```python
from build123d import *

# Parameters (mm, degrees)
F0_W      = 10
F0_H      = 14
F1_DEPTH  = 3
F2_W      = 7
F2_H      = 28
F3_DEPTH  = 35.5
F5_DEPTH  = 70.001
F6_R      = 11.075
F7_DEPTH  = 7
F9_DEPTH  = 25
F10_R     = 2
F11_DEPTH = 2


with BuildPart() as f1:
    # F0 (on Top) → F1 (new body)
    with BuildSketch(Plane.XY):
        with BuildLine():
            ThreePointArc((25, 23), (24.4142135624, 24.4142135624), (23, 25))
            Line((23, 25), (-23, 25))
            ThreePointArc((-23, 25), (-24.4142135624, 24.4142135624), (-25, 23))
            Line((-25, 23), (-25, 14))
            Line((-25, 14), (-25, 0))
            Line((-25, 0), (-25, -14))
            Line((-25, -14), (-25, -23))
            ThreePointArc((-25, -23), (-24.4142135624, -24.4142135624), (-23, -25))
            Line((-23, -25), (23, -25))
            ThreePointArc((23, -25), (24.4142135624, -24.4142135624), (25, -23))
            Line((25, -23), (25, -14))
            Line((25, -14), (25, 0))
            Line((25, 0), (25, 14))
            Line((25, 14), (25, 23))
        make_face()
        with BuildLine():
            ThreePointArc((-20, 18.4), (-21.1313708499, 21.1313708499), (-18.4, 20))
            Line((-18.4, 20), (18.4, 20))
            ThreePointArc((18.4, 20), (20, 21.6), (21.6, 20))
            ThreePointArc((21.6, 20), (21.1313708499, 18.8686291501), (20, 18.4))
            Line((20, 18.4), (20, -18.4))
            ThreePointArc((20, -18.4), (21.1313708499, -18.8686291501), (21.6, -20))
            ThreePointArc((21.6, -20), (20, -21.6), (18.4, -20))
            Line((18.4, -20), (-18.4, -20))
            ThreePointArc((-18.4, -20), (-21.1313708499, -21.1313708499), (-20, -18.4))
            Line((-20, -18.4), (-20, 18.4))
        make_face(mode=Mode.SUBTRACT)
        with Locations((30, 7)):
            Rectangle(F0_W, F0_H)
        with Locations((-30, 7)):
            Rectangle(F0_W, F0_H)
        with Locations((30, -7)):
            Rectangle(F0_W, F0_H)
        with Locations((-30, -7)):
            Rectangle(F0_W, F0_H)
        with BuildLine():
            Line((18.4, 20), (-18.4, 20))
            ThreePointArc((-18.4, 20), (-18.8686291501, 18.8686291501), (-20, 18.4))
            Line((-20, 18.4), (-20, -18.4))
            ThreePointArc((-20, -18.4), (-18.8686291501, -18.8686291501), (-18.4, -20))
            Line((-18.4, -20), (18.4, -20))
            ThreePointArc((18.4, -20), (18.8686291501, -18.8686291501), (20, -18.4))
            Line((20, -18.4), (20, 18.4))
            ThreePointArc((20, 18.4), (18.8686291501, 18.8686291501), (18.4, 20))
        make_face()
    extrude(amount=F1_DEPTH)

    # F2 (on face) → F3 (join)
    with BuildSketch(Plane.XY.offset(3)):
        with Locations((-31.5, 0)):
            Rectangle(F2_W, F2_H)
        with Locations((31.5, 0)):
            Rectangle(F2_W, F2_H)
    extrude(amount=F3_DEPTH)

    # F4 (on face) → F5 (cut, through all)
    with BuildSketch(Plane(origin=(-35, 0, 0), x_dir=(0, -1, 0), z_dir=(-1, 0, 0))):
        with BuildLine():
            Line((14, 38.5), (0, 38.5))
            ThreePointArc((0, 38.5), (9.8994949366, 34.3994949366), (14, 24.5))
            Line((14, 24.5), (14, 38.5))
        make_face()
        with BuildLine():
            ThreePointArc((-14, 24.5), (-9.8994949366, 34.3994949366), (0, 38.5))
            Line((0, 38.5), (-14, 38.5))
            Line((-14, 38.5), (-14, 24.5))
        make_face()
    extrude(amount=-F5_DEPTH, mode=Mode.SUBTRACT)

    # F6 (on face) → F7 (cut, through all)
    with BuildSketch(Plane.YZ.offset(35)):
        with Locations((0, 24.5)):
            Circle(F6_R)
    extrude(amount=-F7_DEPTH, mode=Mode.SUBTRACT)

    # F8 (on face) → F9 (cut)
    with BuildSketch(Plane(origin=(-35, 0, 0), x_dir=(0, -1, 0), z_dir=(-1, 0, 0))):
        with BuildLine():
            ThreePointArc((1, 32), (0.7071067812, 32.7071067812), (0, 33))
            Line((0, 33), (0, 32))
            ThreePointArc((0, 32), (0.5, 31.9833147735), (0.9977753031, 31.9333333333))
            ThreePointArc((0.9977753031, 31.9333333333), (0.999443671, 31.966648112), (1, 32))
        make_face()
        with BuildLine():
            Line((0, 32), (0, 33))
            ThreePointArc((0, 33), (-0.7302967433, 32.6831300511), (-0.9977753031, 31.9333333333))
            ThreePointArc((-0.9977753031, 31.9333333333), (-0.5, 31.9833147735), (0, 32))
        make_face()
        with BuildLine():
            Line((0, 31), (0, 32))
            ThreePointArc((0, 32), (-0.5, 31.9833147735), (-0.9977753031, 31.9333333333))
            ThreePointArc((-0.9977753031, 31.9333333333), (-0.6831300511, 31.2697032567), (0, 31))
        make_face()
        with BuildLine():
            ThreePointArc((0.9977753031, 31.9333333333), (0.5, 31.9833147735), (0, 32))
            Line((0, 32), (0, 31))
            ThreePointArc((0, 31), (0.6831300511, 31.2697032567), (0.9977753031, 31.9333333333))
        make_face()
        with BuildLine():
            ThreePointArc((-6.5, 24.5), (-6.7697032567, 25.1831300511), (-7.4333333333, 25.4977753031))
            ThreePointArc((-7.4333333333, 25.4977753031), (-7.4833147735, 25), (-7.5, 24.5))
            Line((-7.5, 24.5), (-6.5, 24.5))
        make_face()
        with BuildLine():
            ThreePointArc((-7.5, 24.5), (-7.4833147735, 25), (-7.4333333333, 25.4977753031))
            ThreePointArc((-7.4333333333, 25.4977753031), (-8.5, 24.5), (-7.4333333333, 23.5022246969))
            ThreePointArc((-7.4333333333, 23.5022246969), (-7.4833147735, 24), (-7.5, 24.5))
        make_face()
        with BuildLine():
            ThreePointArc((8.5, 24.5), (8.1831300511, 25.2302967433), (7.4333333333, 25.4977753031))
            ThreePointArc((7.4333333333, 25.4977753031), (7.4833147735, 25), (7.5, 24.5))
            ThreePointArc((7.5, 24.5), (7.4833147735, 24), (7.4333333333, 23.5022246969))
            ThreePointArc((7.4333333333, 23.5022246969), (8.1831300511, 23.7697032567), (8.5, 24.5))
        make_face()
        with BuildLine():
            ThreePointArc((7.5, 24.5), (7.4833147735, 25), (7.4333333333, 25.4977753031))
            ThreePointArc((7.4333333333, 25.4977753031), (6.7697032567, 25.1831300511), (6.5, 24.5))
            Line((6.5, 24.5), (7.5, 24.5))
        make_face()
        with BuildLine():
            ThreePointArc((3.75, 24.5), (2.6516504294, 27.1516504294), (0, 28.25))
            Line((0, 28.25), (0, 24.5))
            Line((0, 24.5), (3.75, 24.5))
        make_face()
        with BuildLine():
            Line((0, 24.5), (0, 28.25))
            ThreePointArc((0, 28.25), (-2.6516504294, 27.1516504294), (-3.75, 24.5))
            Line((-3.75, 24.5), (0, 24.5))
        make_face()
        with BuildLine():
            Line((-6.5, 24.5), (-7.5, 24.5))
            ThreePointArc((-7.5, 24.5), (-7.4833147735, 24), (-7.4333333333, 23.5022246969))
            ThreePointArc((-7.4333333333, 23.5022246969), (-6.7697032567, 23.8168699489), (-6.5, 24.5))
        make_face()
        with BuildLine():
            ThreePointArc((7.4333333333, 23.5022246969), (7.4833147735, 24), (7.5, 24.5))
            Line((7.5, 24.5), (6.5, 24.5))
            ThreePointArc((6.5, 24.5), (6.7697032567, 23.8168699489), (7.4333333333, 23.5022246969))
        make_face()
        with BuildLine():
            Line((3.75, 24.5), (0, 24.5))
            Line((0, 24.5), (0, 20.75))
            ThreePointArc((0, 20.75), (2.6516504294, 21.8483495706), (3.75, 24.5))
        make_face()
        with BuildLine():
            Line((0, 20.75), (0, 24.5))
            Line((0, 24.5), (-3.75, 24.5))
            ThreePointArc((-3.75, 24.5), (-2.6516504294, 21.8483495706), (0, 20.75))
        make_face()
        with BuildLine():
            ThreePointArc((0, 18), (-0.6831300511, 17.7302967433), (-0.9977753031, 17.0666666667))
            ThreePointArc((-0.9977753031, 17.0666666667), (-0.5, 17.0166852265), (0, 17))
            Line((0, 17), (0, 18))
        make_face()
        with BuildLine():
            ThreePointArc((0, 17), (-0.5, 17.0166852265), (-0.9977753031, 17.0666666667))
            ThreePointArc((-0.9977753031, 17.0666666667), (-0.033351888, 16.000556329), (1, 17))
            ThreePointArc((1, 17), (0.999443671, 17.033351888), (0.9977753031, 17.0666666667))
            ThreePointArc((0.9977753031, 17.0666666667), (0.5, 17.0166852265), (0, 17))
        make_face()
        with BuildLine():
            Line((0, 18), (0, 17))
            ThreePointArc((0, 17), (0.5, 17.0166852265), (0.9977753031, 17.0666666667))
            ThreePointArc((0.9977753031, 17.0666666667), (0.6831300511, 17.7302967433), (0, 18))
        make_face()
    extrude(amount=-F9_DEPTH, mode=Mode.SUBTRACT)

    # F10 (on face) → F11 (cut)
    with BuildSketch(Plane.YZ.offset(-28)):
        with Locations((-7.5, 24.5)):
            Circle(F10_R)
        with Locations((0, 17)):
            Circle(F10_R)
        with Locations((0, 32)):
            Circle(F10_R)
        with Locations((7.5, 24.5)):
            Circle(F10_R)
    extrude(amount=-F11_DEPTH, mode=Mode.SUBTRACT)


solid = f1.part
```
Here's how the part is built. I have some questions about the finished solid (model axes, mm). A direction names the side the tool comes from. Coordinates: 2 decimals unless noted, no trailing zeros. Order: outer loops, then holes, each group sorted by start corner. A loop starts at its lowest first (then second) coordinate and runs counter-clockwise, first axis right, second up.
1) We'd pull the mould along X, two halves only. Please class faces 6 (the face through (-31, -14, 12)), 7 (the face through (-30, -6.6, 23.6)), 8 (the face through (-28, -0.2, 20.5)): +X half, -X half, draft (parallel to the pull), parting line (faces both ways), or undercut.
2) Which directions (+Z, -Z, +X, -X, +Y, -Y) give clear straight access to the entire face, cutting with the end or side of a thin tool? Please do faces 1 (the face through (-25, 19, 1)), 2 (the face through (31, -14, 12)), 3 (the face through (28, 0, 13)), 4 (the face through (-29, 0, 30)), 5 (the face through (-25, -18, 1)).
3) Will these pins go through, and if not, where does the flat tip stop? pin 1 (1.9 mm diameter, centred on x = -20, y = 20, fed in from +Z); pin 2 (2.5 mm diameter, centred on y = 17.5, z = 1.5, fed in from -X); pin 3 (4.5 mm diameter, centred on y = 0.5, z = 17, fed in from +X); pin 4 (11 mm diameter, centred on x = 32.5, z = 13, fed in from +Y).
4) I need wall thicknesses on line 1 (X direction, y = -20, z = 2); line 2 (X direction, y = 5, z = 4); line 3 (Y direction, x = -29, z = 24). Which ranges of each line are inside material? Lowest first, please.
5) Imagine slicing it at A-A on y = 12. List the corners of the cut face in (x, z) for me.
6) Imagine slicing it at B-B on y = -16. List the corners of the cut face in (x, z) for me.
Response values:
1. face 6: draft
1. face 7: +X half
1. face 8: undercut
2. face 1: +Z, -Z, -X, +Y
2. face 2: +Z, -Z, +X, -Y
2. face 3: +Z, +Y, -Y
2. face 4: +X
2. face 5: +Z, -Z, -X, -Y
3. pin 1: passes through
3. pin 2: stops at x = -25
3. pin 3: stops at x = -28
3. pin 4: stops at y = 14
4. line 1: x = -25 to -21.6, -18.4 to 18.4, 21.6 to 25
4. line 2: x = -35 to -28, 28 to 35
4. line 3: y = -14 to -9.44, -5.56 to -3.72, 3.72 to 5.56, 9.44 to 14
5. outline: (-35, 0) - (35, 0) - (35, 31.71) - (28, 31.71) - (28, 3) - (-28, 3) - (-28, 31.71) - (-35, 31.71) - close
6. outline: (-25, 0) - (25, 0) - (25, 3) - (-25, 3) - close
